Autodesk Inventor part; units mm, degrees
ref_plane "YZ Plane" through (0, 0, 0) normal (1, 0, 0) x (0, 1, 0)
ref_plane "XZ Plane" through (0, 0, 0) normal (0, 1, 0) x (-1, 0, 0)
ref_plane "XY Plane" through (0, 0, 0) normal (0, 0, 1) x (1, 0, 0)
sketch "Sketch1" plane through (0, 0, 0) normal (0, 0, 1) x (1, 0, 0)
  line L0 (0, 0) -> (46, 0)
  line L1 (46, 0) -> (46, 22)
  line L2 (46, 22) -> (0, 22)
  line L3 (0, 22) -> (0, 0)
  dimension "d0" = 46
  dimension "d1" = 22
extrude "Extrusion1" add sketch "Sketch1" along normal blind 5
sketch "Sketch2" plane through (0, 0, 5) normal (0, 0, 1) x (1, 0, 0)
  line L0 (0, 0) -> (46, 0)
  line L1 (46, 0) -> (46, 22)
  circle A0 centre (11.5, 11) radius 8
  circle A1 centre (34.5, 11) radius 8
  point P0 (23, 0)
  point P1 (23, 21.9141)
  point P2 (23, 11)
  point P3 (0, 11)
  point P4 (46, 11)
  dimension "d4" = 16
  dimension "d5" = 16
extrude "Extrusion2" add sketch "Sketch2" along normal blind 10
sketch "Sketch3" plane through (11.5, 11, 15) normal (0, 0, 1) x (1, 0, 0)
  circle A0 centre (0, 0) radius 7
  point P0 (-11.5, -11)
  dimension "d8" = 14
sketch "Sketch4" plane through (34.5, 11, 15) normal (0, 0, 1) x (1, 0, 0)
  circle A0 centre (0, 0) radius 7
  point P0 (-34.5, -11)
  dimension "d9" = 14
extrude "Extrusion3" cut sketch "Sketch3" against normal blind 4
extrude "Extrusion4" cut sketch "Sketch4" against normal blind 4
sketch "Sketch5" plane through (11.5, 11, 11) normal (0, 0, 1) x (1, 0, 0)
  point P0 (-11.5, -11)
sketch "Sketch6" plane through (0, 0, 5) normal (0, 0, 1) x (1, 0, 0)
  point P0 (0, 0)
properties part number "ir sensor" material "Titanium"
CAD build for the part. Positions are in the model's coordinates, mm. A direction names the side the tool comes from. Round coordinates to 2 decimals unless told otherwise and drop trailing zeros. Write each loop counter-clockwise with the first axis right and the second up, starting at its lowest first coordinate (ties: lowest second). Pieces come first, ordered by that corner, then holes.
(1) Slice it at C-C, the plane x = 34.5. Write the cut outline in (y, z), and give its area (3 significant figures).
(2) Slice it at A-A, the plane z = 12.25. Write the cut outline in (x, y), and give its area (3 significant figures).
(3) Slice it at D-D, the plane y = 8. Write the cut outline in (x, z), and give its area (3 significant figures).
(4) 3-axis set-ups, long thin cutter, end or side, ignore diameter. For faces 1 (the face through (28.151, 15.868, 9.93)), 2 (the face through (23, 22, 2)): which of +Z, -Z, +X, -X, +Y, -Y reach the whole face in a straight line?
(5) Probe line 1 along Y through (x, z) = (11.5, 12.75); line 2 along Z through (x, y) = (14.5, 6.25); line 3 along Z through (x, y) = (5, 4.25). List the from-to ranges inside material, lowest first.
(6) Slice it at B-B, the plane y = 11. Write the cut outline in (x, z).
(7) Mould opens along X. For faces 3 (the face through (0, 11, 2)), 4 (the face through (23, 11, 5)), 5 (the face through (23, 11, 0)), 6 (the face through (14.73, 4.79, 13.03)) say: pulls with the +X half, pulls with the -X half, needs draft (parallel to the pull), parting line crosses it, or undercut.
(8) Drop flat-ended pins along their axis: P1, Ø1, axis at x = 20.5, z = 8.5, coming from the -Y side; P2, Ø1, axis at x = 27, y = 4.5, coming from the +Z side; P3, Ø3, axis at y = 7, z = 9, coming from the +X side; P4, Ø12.5, axis at x = 11.5, y = 11, coming from the +Z side. Give the stop position or say it passes through.
From the geometry:
1. outline: (0, 0) - (22, 0) - (22, 5) - (19, 5) - (19, 15) - (18, 15) - (18, 11) - (4, 11) - (4, 15) - (3, 15) - (3, 5) - (0, 5) - close
1. area: 214 mm2
2. outline: circle Ø16 at (11.5, 11); circle Ø16 at (34.5, 11); hole circle Ø14 at (11.5, 11); hole circle Ø14 at (34.5, 11)
2. area: 94.2 mm2
3. outline: (0, 0) - (46, 0) - (46, 5) - (41.92, 5) - (41.92, 15) - (40.82, 15) - (40.82, 11) - (28.18, 11) - (28.18, 15) - (27.08, 15) - (27.08, 5) - (18.92, 5) - (18.92, 15) - (17.82, 15) - (17.82, 11) - (5.18, 11) - (5.18, 15) - (4.08, 15) - (4.08, 5) - (0, 5) - close
3. area: 425 mm2
4. face 1: +Z
4. face 2: +Z, -Z, +X, -X, +Y
5. line 1: y = 3 to 4, 18 to 19
5. line 2: z = 0 to 11
5. line 3: z = 0 to 5
6. outline: (0, 0) - (46, 0) - (46, 5) - (42.5, 5) - (42.5, 15) - (41.5, 15) - (41.5, 11) - (27.5, 11) - (27.5, 15) - (26.5, 15) - (26.5, 5) - (19.5, 5) - (19.5, 15) - (18.5, 15) - (18.5, 11) - (4.5, 11) - (4.5, 15) - (3.5, 15) - (3.5, 5) - (0, 5) - close
7. face 3: pulls with the -X half
7. face 4: undercut
7. face 5: needs draft
7. face 6: undercut
8. P1: passes through
8. P2: stops at z = 5
8. P3: stops at x = 42.1
8. P4: stops at z = 11
